from build123d import *

# Parameters (mm, degrees)
SKIZZE1_R       = 1.5
BASE_DEPTH      = 2.5
SKIZZE3_W       = 21.742814906
SKIZZE3_H       = 7.5
SKIZZE3_R       = 1.5
DISTANCER_DEPTH = 0.3


with BuildPart() as part:
    # Skizze1 → Base (new body)
    with BuildSketch(Plane.XY):
        with BuildLine():
            Line((-15, 3.75), (15, 3.75))
            ThreePointArc((15, 3.75), (18.75, 0), (15, -3.75))
            Line((15, -3.75), (-15, -3.75))
            ThreePointArc((-15, -3.75), (-18.75, 0), (-15, 3.75))
        make_face()
        with Locations((-15, 0)):
            Circle(SKIZZE1_R, mode=Mode.SUBTRACT)
        with Locations((15, 0)):
            Circle(SKIZZE1_R, mode=Mode.SUBTRACT)
        with Locations((-8, 0)):
            Circle(SKIZZE1_R, mode=Mode.SUBTRACT)
        with Locations((8, 0)):
            Circle(SKIZZE1_R, mode=Mode.SUBTRACT)
    extrude(amount=BASE_DEPTH)

    # Skizze3 → Distancer (add)
    # profile 1 of 3: a face of its own
    with BuildSketch(Plane.XY.offset(2.5)):
        with BuildLine():
            ThreePointArc((-10.871407453, 3.75), (-11.5, 0), (-10.871407453, -3.75))
            Line((-10.871407453, -3.75), (-10.871407453, 3.75))
        make_face()
    # profile 2 of 3: a face of its own
    with BuildSketch(Plane.XY.offset(2.5)):
        with BuildLine():
            Line((10.871407453, 3.75), (10.871407453, -3.75))
            ThreePointArc((10.871407453, -3.75), (11.341763216, -1.901159422), (11.5, 0))
            ThreePointArc((11.5, 0), (11.341763216, 1.901159422), (10.871407453, 3.75))
        make_face()
    # profile 3 of 3: a face of its own
    with BuildSketch(Plane.XY.offset(2.5)):
        Rectangle(SKIZZE3_W, SKIZZE3_H)
        with Locations((-8, 0)):
            Circle(SKIZZE3_R, mode=Mode.SUBTRACT)
        with Locations((8, 0)):
            Circle(SKIZZE3_R, mode=Mode.SUBTRACT)
    extrude(amount=DISTANCER_DEPTH)


solid = part.part
Can you work these out from the model? Positions are in its coordinate system, mm. Round coordinates to 2 decimals unless told otherwise and drop trailing zeros. Order: outer loops, then holes, each group sorted by start corner. A loop starts at its lowest first (then second) coordinate and runs counter-clockwise, first axis right, second up. Notation, with made-up numbers: (-23.5, 58.5) - (4.5, 58.5) arc R28 cw to (4.5, 77.5) - close; hole circle Ø9 at (-34.5, 43). An arc over 180 degrees is marked (long way). Answer in a Markdown table with one row per item.
(1) Suppose I cut it at B-B, the plane z = 1.65. Please give me the cut outline in (x, y).
From the geometry:
| item | result |
|---|---|
| outline | (-15, -3.75) - (15, -3.75) arc R3.75 ccw to (15, 3.75) - (-15, 3.75) arc R3.75 ccw to start; hole circle Ø3 at (-15, 0); hole circle Ø3 at (-8, 0); hole circle Ø3 at (8, 0); hole circle Ø3 at (15, 0) |
(2) Suppose I cut it at D-D, the plane y = -2.5. Please give me the cut outline in (x, z), plus the area to 3 significant figures.
From the geometry:
| item | result |
|---|---|
| outline | (-17.8, 0) - (17.8, 0) - (17.8, 2.5) - (11.22, 2.5) - (11.22, 2.8) - (-11.22, 2.8) - (-11.22, 2.5) - (-17.8, 2.5) - close |
| area | 95.7 mm2 |
(3) Suppose I cut it at A-A, the plane x = 8. Please give me the cut outline in (y, z).
From the geometry:
| item | result |
|---|---|
| outline | (-3.75, 0) - (-1.5, 0) - (-1.5, 2.8) - (-3.75, 2.8) - close; (1.5, 0) - (3.75, 0) - (3.75, 2.8) - (1.5, 2.8) - close |
(4) For P1, Ø4, axis at x = -16, y = -1.5, coming from the +Z side, with a flat end and sliding along its axis, tell me the tip position at first contact or that it passes through.
From the geometry:
| item | result |
|---|---|
| P1 | stops at z = 2.5 |
(5) Please list where these lines run through material, in increasing order: L1, parallel to Y at x = 15, z = 1.9; L2, parallel to X at y = 1, z = 1.6; L3, parallel to X at y = 0.25, z = 0.15. Write a range as from..to.
From the geometry:
| item | result |
|---|---|
| L1 | y = -3.75..-1.5, 1.5..3.75 |
| L2 | x = -18.61..-16.12, -13.88..-9.12, -6.88..6.88, 9.12..13.88, 16.12..18.61 |
| L3 | x = -18.74..-16.48, -13.52..-9.48, -6.52..6.52, 9.48..13.52, 16.48..18.74 |
(6) If we mould it in two halves opening along Y, with no side actions, what happens to faces 1 (the face through (-15, -2, 2.5)), 2 (the face through (18.75, 0.08, 1.23)), 3 (the face through (-9.5, 0.07, 1.38)), 4 (the face through (6.5, 0.07, 1.38))? For each: released by +Y, released by -Y, zero draft, split by the parting line, or undercut.
From the geometry:
| item | result |
|---|---|
| face 1 | zero draft |
| face 2 | split by the parting line |
| face 3 | undercut |
| face 4 | undercut |
(7) Suppose I cut it at C-C, the plane y = 0.75. Please give me the cut outline in (x, z), plus the area to 3 significant figures.
From the geometry:
| item | result |
|---|---|
| outline | (-18.67, 0) - (-16.3, 0) - (-16.3, 2.5) - (-18.67, 2.5) - close; (-13.7, 0) - (-9.3, 0) - (-9.3, 2.8) - (-11.48, 2.8) - (-11.48, 2.5) - (-13.7, 2.5) - close; (-6.7, 0) - (6.7, 0) - (6.7, 2.8) - (-6.7, 2.8) - close; (9.3, 0) - (13.7, 0) - (13.7, 2.5) - (11.48, 2.5) - (11.48, 2.8) - (9.3, 2.8) - close; (16.3, 0) - (18.67, 0) - (18.67, 2.5) - (16.3, 2.5) - close |
| area | 72.7 mm2 |
